Could you check a few things on this drawing? It's one solid part, dimensions in mm from its lowest x, y, z. A direction names the side the tool comes from. Coordinates: 2 decimals unless noted, no trailing zeros. Order: outer loops, then holes, each group sorted by start corner. A loop starts at its lowest first (then second) coordinate and runs counter-clockwise, first axis right, second up. Notation, with made-up numbers: M 82,47.25 L 124,47.25 A15 cw 124,72.25 Z; hole C 88.25,69.5 d8. An arc over 180 degrees is marked long. Write item = value, one per line. Start each with the question number.
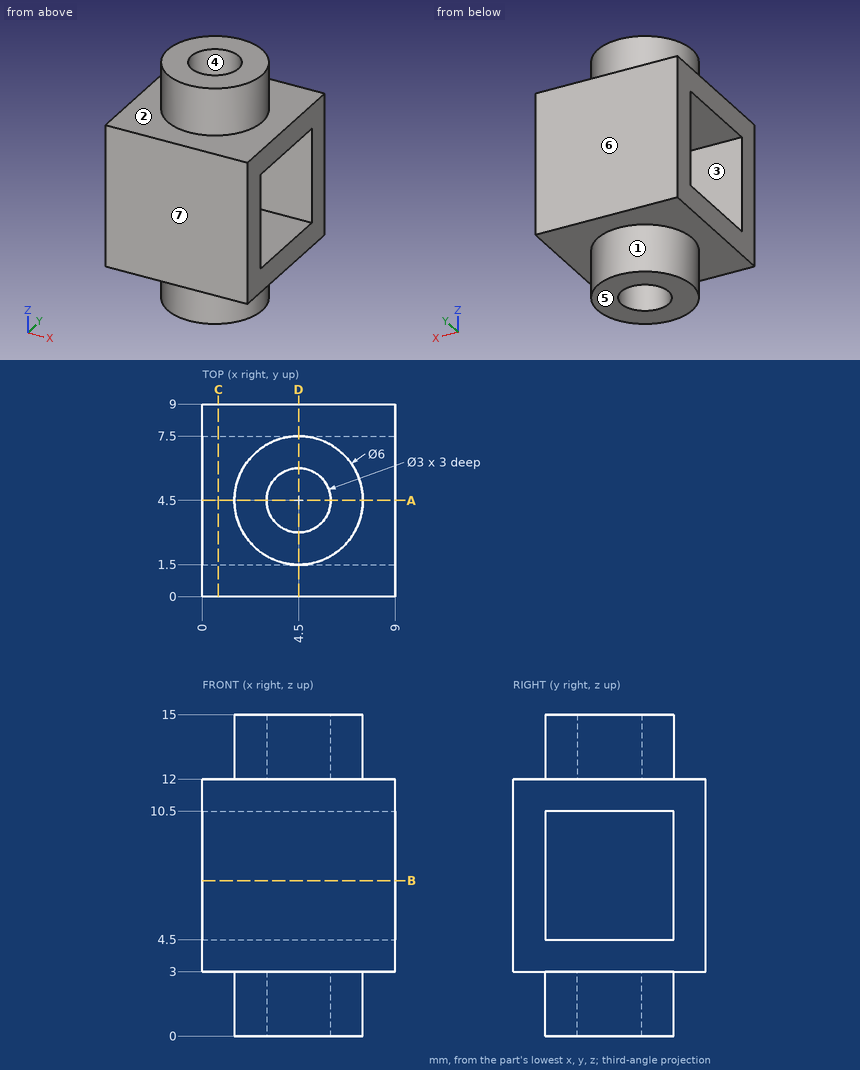
(1) Thinking about a two-plate mould opening in Y: for the marked faces 4, 5, 6 and 7, which applies, released by +Y, released by -Y, zero draft, split by the parting line, or undercut?
(2) Imagine slicing it at C-C on x = 0.75. List the corners of the cut face in (y, z) for me, plus the area to 3 significant figures.
(3) Imagine slicing it at D-D on x = 4.5. List the corners of the cut face in (y, z) for me, plus the area to 3 significant figures.
(4) For the marked faces 1, 2 and 3, which set-ups out of +Z, -Z, +X, -X, +Y, -Y let a thin tool reach every point of the face, with its end or its side?
(5) Please list where these lines run through material, in increasing order: probe 1 along Z at (x, y) = (1.5, 6.75); probe 2 along Y at (x, z) = (4.5, 13); probe 3 along Z at (x, y) = (3.5, 6.5). Write a range as from..to.
(6) Imagine slicing it at A-A on y = 4.5. List the corners of the cut face in (x, z) for me.
(7) Will these pins go through, and if not, where does the flat tip stop? P1, Ø4, axis at x = 5, y = 7, coming from the -Z side; P2, Ø1.5, axis at x = 4.5, y = 5, coming from the -Z side; P3, Ø0.9, axis at x = 5, y = 4.5, coming from the +Z side.
(8) Imagine slicing it at B-B on z = 7.25. List the corners of the cut face in (x, y) for me.
Response:
q1.face_4 = undercut
q1.face_5 = zero draft
q1.face_6 = released by +Y
q1.face_7 = released by -Y
q2.outline = M 0,3 L 9,3 L 9,12 L 0,12 Z; hole M 1.5,4.5 L 7.5,4.5 L 7.5,10.5 L 1.5,10.5 Z
q2.area = 45.0 mm2
q3.outline = M 0,3 L 1.5,3 L 1.5,0 L 3,0 L 3,3 L 6,3 L 6,0 L 7.5,0 L 7.5,3 L 9,3 L 9,12 L 7.5,12 L 7.5,15 L 6,15 L 6,12 L 3,12 L 3,15 L 1.5,15 L 1.5,12 L 0,12 Z; hole M 1.5,4.5 L 7.5,4.5 L 7.5,10.5 L 1.5,10.5 Z
q3.area = 63.0 mm2
q4.face_1 = -Z
q4.face_2 = +Z
q4.face_3 = +X, -X
q5.probe_1 = 3..4.5, 10.5..12
q5.probe_2 = 1.5..3, 6..7.5
q5.probe_3 = 0..4.5, 10.5..15
q6.outline = M 0,3 L 1.5,3 L 1.5,0 L 3,0 L 3,3 L 6,3 L 6,0 L 7.5,0 L 7.5,3 L 9,3 L 9,4.5 L 0,4.5 Z; M 0,10.5 L 9,10.5 L 9,12 L 7.5,12 L 7.5,15 L 6,15 L 6,12 L 3,12 L 3,15 L 1.5,15 L 1.5,12 L 0,12 Z
q7.P1 = 0
q7.P2 = 3
q7.P3 = 12
q8.outline = M 0,0 L 9,0 L 9,1.5 L 0,1.5 Z; M 0,7.5 L 9,7.5 L 9,9 L 0,9 Z
